The listing builds one solid part. Answer for the finished solid, in the listing's coordinates (mm). A direction names the side the tool comes from. Coordinates: 2 decimals unless noted, no trailing zeros. Order: outer loops, then holes, each group sorted by start corner. A loop starts at its lowest first (then second) coordinate and runs counter-clockwise, first axis right, second up. Notation, with made-up numbers: (50.5, 1.25) - (98.5, 1.25) arc R32 ccw to (98.5, 32.25) - close; hole circle Ø5 at (-14.5, -27). An arc over 180 degrees is marked (long way). One line per item, written item: value. Start each with the question number.
Autodesk Inventor part; units mm, degrees
ref_plane "YZ Plane" through (0, 0, 0) normal (1, 0, 0) x (0, 1, 0)
ref_plane "XZ Plane" through (0, 0, 0) normal (0, 1, 0) x (-1, 0, 0)
ref_plane "XY Plane" through (0, 0, 0) normal (0, 0, 1) x (1, 0, 0)
sketch "Skizze1" plane through (0, 0, 0) normal (1, 0, 0) x (0, 1, 0)
  line L0 (0, 0) -> (144, 0)
  line L1 (144, 0) -> (144, -68)
  line L2 (144, -68) -> (0, -68)
  line L3 (0, -68) -> (0, 0)
  dimension "d0" = 144
  dimension "d1" = 68
extrude "Extrusion1" add sketch "Skizze1" along normal blind 16
sketch "Skizze2" plane through (0, 0, 0) normal (0, 0, 1) x (1, 0, 0)
  line L0 (0, 0) -> (0, 144) construction
  line L1 (0, 72) -> (16, 72) construction
  line L2 (16, 144) -> (16, 0) construction
  line L3 (0, 144) -> (16, 144) construction
  line L4 (8, 144) -> (8, 0) construction
  line L5 (0, 144) -> (16, 144) construction
  line L6 (0, 0) -> (16, 0) construction
  line L7 (0, 144) -> (16, 144) construction
  line L8 (16, 144) -> (16, 0) construction
  line L9 (16, 0) -> (0, 0) construction
  line L10 (0, 0) -> (0, 144) construction
  line L11 (0, 112) -> (16, 112) construction
  line L12 (0, 32) -> (16, 32) construction
  point P0 (8, 112)
  point P1 (8, 72)
  point P2 (8, 32)
  dimension "d4" = 40
  dimension "d5" = 40
hole "Bohrung1" at (8, 112, 0) at (8, 72, 0) at (8, 32, 0) direction (0, 0, -1) diameter 3 depth 30 tip angle 118
sketch "Skizze3" plane through (0, 144, 0) normal (0, 1, 0) x (1, 0, 0)
  line L0 (0, 0) -> (16, 0)
  line L1 (16, 0) -> (16, 68)
  line L2 (16, 68) -> (0, 68)
  line L3 (0, 68) -> (0, 0)
  line L4 (8, 0) -> (8, 68) construction
  line L5 (0, 68) -> (16, 68) construction
  line L6 (16, 0) -> (16, 68) construction
  line L7 (16, 34) -> (0, 34) construction
  line L8 (0, 68) -> (0, 0) construction
  line L9 (0, 14) -> (16, 14) construction
  line L10 (0, 54) -> (16, 54) construction
  point P0 (8, 14)
  point P1 (8, 54)
  dimension "d13" = 14
  dimension "d22" = 14
hole "Bohrung2" at (8, 144, -14) at (8, 144, -54) direction (0, -1, 0) diameter 3 depth 25 tip angle 118
sketch "Skizze4" plane through (0, 0, -68) normal (0, 0, -1) x (-1, 0, 0)
  line L0 (0, 0) -> (-16, 0) construction
  line L1 (-16, 0) -> (-16, 144) construction
  line L2 (-16, 144) -> (0, 144) construction
  line L3 (0, 144) -> (0, 0) construction
  line L4 (-8, 0) -> (-8, 144) construction
  line L5 (-16, 144) -> (-16, 0) construction
  line L6 (-16, 72) -> (0, 72) construction
  circle A0 centre (-8, 72) radius 1.5 construction
  point P0 (-8, 112)
  point P1 (-8, 32)
  dimension "d23" = 40
  dimension "d24" = 40
hole "Bohrung3" at (8, 72, -68) at (8, 112, -68) at (8, 32, -68) direction (0, 0, 1) diameter 3 depth 30 tip angle 118
sketch "Skizze5" plane through (16, 0, 0) normal (1, 0, 0) x (0, 0, -1)
  line L0 (0, 0) -> (68, 0) construction
  line L1 (68, 0) -> (68, 144) construction
  line L2 (68, 144) -> (0, 144) construction
  line L3 (0, 144) -> (0, 0) construction
  line L4 (0, 0) -> (68, 0) construction
  line L5 (34, 0) -> (34, 144) construction
  line L6 (0, 72) -> (68, 72) construction
  line L7 (68, 73.5) -> (68, 70.5) construction
  point P0 (34, 52)
  point P1 (34, 92)
  dimension "d32" = 20
  dimension "d33" = 20
hole "Bohrung4" at (16, 52, -34) at (16, 92, -34) direction (-1, 0, 0) diameter 24 end through all
equation "\"d39\" = Stärke"
equation "\"Biegeradius\" = Stärke"
equation "\"BreiteBiegungsfreistellung\" = Stärke"
equation "\"TiefeBiegungsfreistellung\" = 0.5 * Stärke"
equation "\"GrößeEckenfreistellung\" = 4 * Stärke"
equation "\"MinimalRest\" = 2 * Stärke"
equation "\"Übergangsradius\" = Biegeradius"
equation "\"JacobiRadiusGröße\" = Biegeradius"
equation "\"Abstandsgröße\" = Stärke"
properties part number "licht_side_200_middle"
(1) Consider probe 1 along Y at (x, z) = (9.5, -34.5); probe 2 along Y at (x, z) = (8, -48); probe 3 along Y at (x, z) = (4.5, -30). Determine where each line is inside the solid, lowest interval first.
(2) For faces 4 (the face through (7.888, 56.596, -45.085)), 5 (the face through (7.93, 110.5, -52.79)), 6 (the face through (9.464, 131.325, -54.325)), 7 (the face through (7.93, 113.5, -15.21)), determine the directions among +Z, -Z, +X, -X, +Y, -Y from which every point of the face is accessible in a straight line to the end or side of a thin tool.
(3) Flat-ended cylindrical pins translate along their axes: pin 1 Ø2.5 at (x, y) = (8, 72) entering from -Z; pin 2 Ø1.8 at (x, y) = (8, 72) entering from +Z; pin 3 Ø1.8 at (x, y) = (8, 112) entering from -Z. Find the tip coordinate at first contact, or state that the pin passes through.
(4) The part is cut by section C-C on x = 2. Determine the outline of the cut face in (y, z), plus the area to 3 significant figures.
(5) The part is cut by section D-D on y = 90. Determine the outline of the cut face in (x, z), plus the area to 3 significant figures.
(6) The part is cut by section B-B on z = -34. Determine the outline of the cut face in (x, y).
(7) For a pull along Y with two mould halves and no side action, classify faces 1 (the face through (8.011, 111.74, -37.255)), 2 (the face through (8.9, 131.3, -15.2)), 3 (the face through (8, 0, -34)) as pulls with the +Y half, pulls with the -Y half, needs draft (parallel to the pull), parting line crosses it, or undercut.
(8) The part is cut by section A-A on y = 52. Determine the outline of the cut face in (x, z).
Completed:
1. probe 1: y = 0 to 40.01, 63.99 to 80.01, 103.99 to 144
1. probe 2: y = 0 to 30.5, 33.5 to 70.5, 73.5 to 110.5, 113.5 to 144
1. probe 3: y = 0 to 40.69, 63.31 to 80.69, 103.31 to 144
2. face 4: +X, -X
2. face 5: -Z
2. face 6: +Y
2. face 7: +Z
3. pin 1: stops at z = -37.85
3. pin 2: stops at z = -30.36
3. pin 3: stops at z = -37.64
4. outline: (0, -68) - (144, -68) - (144, 0) - (0, 0) - close; hole circle Ø24 at (52, -34); hole circle Ø24 at (92, -34)
4. area: 8,890 mm2
5. outline: (0, -68) - (16, -68) - (16, -45.83) - (0, -45.83) - close; (0, -22.17) - (16, -22.17) - (16, 0) - (0, 0) - close
5. area: 709 mm2
6. outline: (0, 0) - (16, 0) - (16, 40) - (0, 40) - close; (0, 64) - (16, 64) - (16, 80) - (0, 80) - close; (0, 104) - (16, 104) - (16, 144) - (0, 144) - close
7. face 1: undercut
7. face 2: needs draft
7. face 3: pulls with the -Y half
8. outline: (0, -68) - (16, -68) - (16, -46) - (0, -46) - close; (0, -22) - (16, -22) - (16, 0) - (0, 0) - close
